Geometry: final body of the model. Coordinates: model frame, mm. A direction names the side the tool comes from. Coordinates: 2 decimals unless noted, no trailing zeros. Loops run counter-clockwise (first coordinate to the right, second up) from the corner with the lowest first, then second, coordinate; pieces in that order, holes last. Notation, with made-up numbers: (26, 21) -> (44, 21) arc R28 cw to (44, 39) -> close; hole circle Ø8 at (-19, 54). An arc over 180 degrees is marked (long way). One line per item, written item: value. Start each with the question number.
Item 1: Ray query, probe 1 along Y at (x, z) = (55, -4.6); probe 2 along Y at (x, z) = (5.5, 6). Return the intervals inside material, ascending. Write a range as from..to.
Item 2: Set-up query: faces 4 (the cylindrical face through (-2.708, 64.086, -13.412)), 5 (the flat face through (-4, 1.5, -13)). Return all of +Z, -Z, +X, -X, +Y, -Y with unobstructed straight access to the full face (end or side cutting, diameter ignored); none if empty.
Item 3: Section query C-C on z = -3. Give the number of separate pieces and of enclosed holes in the cut face, then the cut area to 3 significant figures.
Item 4: Mould query, pull axis Y, two halves, no side actions, for faces 1 (the cylindrical face through (56.6, 30.1, -8.2)), 2 (the flat face through (30, -7.5, -5)), 3 (the flat face through (55, 55, -16.37)). Classes: +Y half, -Y half, draft (parallel to the pull), parting line (faces both ways), or undercut.
Item 5: Contact query for flat-ended pins moving along their axis: pin 1 Ø1 at (x, z) = (64, -13) entering from -Y; pin 2 Ø4.5 at (x, y) = (54, 55.5) entering from +Z; pin 3 Ø1.8 at (x, z) = (-5, -13) entering from +Y; pin 4 Ø5 at (x, z) = (64, -8) entering from +Y. Output: stop coordinate, or through.
Item 6: Section query D-D on z = 2.5. Return loops of the section in (x, y), then the cut area to 3 significant figures.
Item 7: Section query A-A on x = 20. Return loops of the section in (y, z), then the cut area to 3 significant figures.
from build123d import *

# Parameters (mm, degrees)
SIDES_START         = -14.970203
SIDES_DEPTH         = 21.970205
BOSS_EXTRUDE2_START = -16.370201
SKETCH1_3_R         = 1.6
BOSS_EXTRUDE2_DEPTH = 1.4
BOSS_EXTRUDE3_START = -16.370203
SKETCH1_4_R         = 1.6
BOSS_EXTRUDE3_DEPTH = 6.000003
BOSS_EXTRUDE4_START = -1.619402
SKETCH1_5_R         = 4.998410694
SKETCH1_5_R_2       = 5.00000078
SKETCH1_5_R_3       = 4.998409474
SKETCH1_5_R_4       = 2
BOSS_EXTRUDE4_DEPTH = 14.75080016
CUT_EXTRUDE1_START  = -7.619402
SKETCH1_6_R         = 2
CUT_EXTRUDE1_DEPTH  = 6
BOSS_EXTRUDE5_START = -1.619402
SKETCH2_R           = 1.6
SKETCH2_W           = 2.2
SKETCH2_H           = 10
BOSS_EXTRUDE5_DEPTH = 13.350799067
BOSS_EXTRUDE6_START = -14.9702
SKETCH2_3_W         = 2.2
SKETCH2_3_H         = 10
BOSS_EXTRUDE6_DEPTH = 19.9702
CUT_EXTRUDE2_START  = -3e-06
CUT_EXTRUDE2_DEPTH  = 23.370208


with BuildPart() as part:
    # Sketch1 → sides (new body)
    with BuildSketch(Plane.XY.offset(SIDES_START)):
        with BuildLine():
            ThreePointArc((-7.5, 62.5), (-6.035533906, 66.035533906), (-2.5, 67.5))
            Line((-2.5, 67.5), (62.5, 67.5))
            ThreePointArc((62.5, 67.5), (66.035533906, 66.035533906), (67.5, 62.5))
            Line((67.5, 62.5), (67.5, -2.5))
            ThreePointArc((67.5, -2.5), (66.035533906, -6.035533906), (62.5, -7.5))
            Line((62.5, -7.5), (-2.5, -7.5))
            ThreePointArc((-2.5, -7.5), (-6.035533906, -6.035533906), (-7.5, -2.5))
            Line((-7.5, -2.5), (-7.5, 62.5))
        make_face()
        with BuildLine():
            ThreePointArc((66, 62.5), (64.974873734, 64.974873734), (62.5, 66))
            Line((62.5, 66), (61, 66))
            Line((61, 66), (-1, 66))
            Line((-1, 66), (-2.5, 66))
            ThreePointArc((-2.5, 66), (-4.974873734, 64.974873734), (-6, 62.5))
            Line((-6, 62.5), (-6, 61.010980342))
            Line((-6, 61.010980342), (-6, -1))
            Line((-6, -1), (-6, -2.5))
            ThreePointArc((-6, -2.5), (-4.974873734, -4.974873734), (-2.5, -6))
            Line((-2.5, -6), (-1, -6))
            Line((-1, -6), (61, -6))
            Line((61, -6), (62.5, -6))
            ThreePointArc((62.5, -6), (64.974873734, -4.974873734), (66, -2.5))
            Line((66, -2.5), (66, -1))
            Line((66, -1), (66, 61.010980342))
            Line((66, 61.010980342), (66, 62.5))
        make_face(mode=Mode.SUBTRACT)
    extrude(amount=SIDES_DEPTH)

    # Sketch1<3> → Boss-Extrude2 (add)
    with BuildSketch(Plane.XY.offset(BOSS_EXTRUDE2_START)):
        with BuildLine():
            Line((67.5, 62.5), (67.5, -2.5))
            ThreePointArc((67.5, -2.5), (66.035533906, -6.035533906), (62.5, -7.5))
            Line((62.5, -7.5), (-2.5, -7.5))
            ThreePointArc((-2.5, -7.5), (-6.035533906, -6.035533906), (-7.5, -2.5))
            Line((-7.5, -2.5), (-7.5, 62.5))
            ThreePointArc((-7.5, 62.5), (-6.035533906, 66.035533906), (-2.5, 67.5))
            Line((-2.5, 67.5), (62.5, 67.5))
            ThreePointArc((62.5, 67.5), (66.035533906, 66.035533906), (67.5, 62.5))
        make_face()
        with Locations((-2.5, 62.5)):
            Circle(SKETCH1_3_R, mode=Mode.SUBTRACT)
        with Locations((62.5, 62.5)):
            Circle(SKETCH1_3_R, mode=Mode.SUBTRACT)
        with Locations((-2.5, -2.5)):
            Circle(SKETCH1_3_R, mode=Mode.SUBTRACT)
        with Locations((62.5, -2.5)):
            Circle(SKETCH1_3_R, mode=Mode.SUBTRACT)
    extrude(amount=BOSS_EXTRUDE2_DEPTH)

    # Sketch1<4> → Boss-Extrude3 (add)
    # profile 1 of 4: a face of its own
    with BuildSketch(Plane.XY.offset(BOSS_EXTRUDE3_START)):
        with BuildLine():
            ThreePointArc((66, 62.5), (64.974873734, 64.974873734), (62.5, 66))
            Line((62.5, 66), (58.5, 66))
            Line((58.5, 66), (58.5, 62.5))
            ThreePointArc((58.5, 62.5), (59.671572875, 59.671572875), (62.5, 58.5))
            Line((62.5, 58.5), (66, 58.5))
            Line((66, 58.5), (66, 62.5))
        make_face()
        with Locations((62.5, 62.5)):
            Circle(SKETCH1_4_R, mode=Mode.SUBTRACT)
    # profile 2 of 4: a face of its own
    with BuildSketch(Plane.XY.offset(BOSS_EXTRUDE3_START)):
        with BuildLine():
            Line((1.5, 62.5), (1.5, 66))
            Line((1.5, 66), (-2.5, 66))
            ThreePointArc((-2.5, 66), (-4.974873734, 64.974873734), (-6, 62.5))
            Line((-6, 62.5), (-6, 58.5))
            Line((-6, 58.5), (-2.5, 58.5))
            ThreePointArc((-2.5, 58.5), (0.328427125, 59.671572875), (1.5, 62.5))
        make_face()
        with Locations((-2.5, 62.5)):
            Circle(SKETCH1_4_R, mode=Mode.SUBTRACT)
    # profile 3 of 4: a face of its own
    with BuildSketch(Plane.XY.offset(BOSS_EXTRUDE3_START)):
        with BuildLine():
            Line((66, -2.5), (66, 1.5))
            Line((66, 1.5), (62.5, 1.5))
            ThreePointArc((62.5, 1.5), (59.671572875, 0.328427125), (58.5, -2.5))
            Line((58.5, -2.5), (58.5, -6))
            Line((58.5, -6), (62.5, -6))
            ThreePointArc((62.5, -6), (64.974873734, -4.974873734), (66, -2.5))
        make_face()
        with Locations((62.5, -2.5)):
            Circle(SKETCH1_4_R, mode=Mode.SUBTRACT)
    # profile 4 of 4: a face of its own
    with BuildSketch(Plane.XY.offset(BOSS_EXTRUDE3_START)):
        with BuildLine():
            Line((-2.5, 1.5), (-6, 1.5))
            Line((-6, 1.5), (-6, -2.5))
            ThreePointArc((-6, -2.5), (-4.974873734, -4.974873734), (-2.5, -6))
            Line((-2.5, -6), (1.5, -6))
            Line((1.5, -6), (1.5, -2.5))
            ThreePointArc((1.5, -2.5), (0.328427125, 0.328427125), (-2.5, 1.5))
        make_face()
        with Locations((-2.5, -2.5)):
            Circle(SKETCH1_4_R, mode=Mode.SUBTRACT)
    extrude(amount=BOSS_EXTRUDE3_DEPTH)

    # Sketch1<5> → Boss-Extrude4 (add)
    with BuildSketch(Plane.XY.offset(BOSS_EXTRUDE4_START)):
        with Locations((55.001589559, 4.998410441)):
            Circle(SKETCH1_5_R)
        with Locations((54.99999922, 54.99999922)):
            Circle(SKETCH1_5_R_2)
        with Locations((5.00000016, 54.99999922)):
            Circle(SKETCH1_5_R_2)
        with Locations((4.998409221, 4.998409221)):
            Circle(SKETCH1_5_R_3)
        with Locations((4.998409221, 4.998409221)):
            Circle(SKETCH1_5_R_4)
        with Locations((55.001589559, 4.998410441)):
            Circle(SKETCH1_5_R_4)
        with Locations((54.99999922, 54.99999922)):
            Circle(SKETCH1_5_R_4)
        with Locations((5.00000016, 54.99999922)):
            Circle(SKETCH1_5_R_4)
    extrude(amount=-BOSS_EXTRUDE4_DEPTH)

    # Sketch1<6> → Cut-Extrude1 (cut)
    with BuildSketch(Plane.XY.offset(CUT_EXTRUDE1_START)):
        with Locations((4.998409221, 4.998409221)):
            Circle(SKETCH1_6_R)
        with Locations((55.001589559, 4.998410441)):
            Circle(SKETCH1_6_R)
        with Locations((54.99999922, 54.99999922)):
            Circle(SKETCH1_6_R)
        with Locations((5.00000016, 54.99999922)):
            Circle(SKETCH1_6_R)
    extrude(amount=CUT_EXTRUDE1_DEPTH, mode=Mode.SUBTRACT)

    # Sketch2 → Boss-Extrude5 (add)
    # profile 1 of 4: a face of its own
    with BuildSketch(Plane.XY.offset(BOSS_EXTRUDE5_START)):
        with BuildLine():
            ThreePointArc((-1.6, 25), (3.4, 30), (-1.6, 35))
            Line((-1.6, 35), (-3.8, 35))
            Line((-3.8, 35), (-3.8, 25))
            Line((-3.8, 25), (-1.6, 25))
        make_face()
        with Locations((-1.6, 30)):
            Circle(SKETCH2_R, mode=Mode.SUBTRACT)
    # profile 2 of 4: a face of its own
    with BuildSketch(Plane.XY.offset(BOSS_EXTRUDE5_START)):
        with Locations((-4.9, 30)):
            Rectangle(SKETCH2_W, SKETCH2_H)
    # profile 3 of 4: a face of its own
    with BuildSketch(Plane.XY.offset(BOSS_EXTRUDE5_START)):
        with BuildLine():
            Line((63.8, 35), (61.6, 35))
            ThreePointArc((61.6, 35), (56.6, 30), (61.6, 25))
            Line((61.6, 25), (63.8, 25))
            Line((63.8, 25), (63.8, 35))
        make_face()
        with Locations((61.6, 30)):
            Circle(SKETCH2_R, mode=Mode.SUBTRACT)
    # profile 4 of 4: a face of its own
    with BuildSketch(Plane.XY.offset(BOSS_EXTRUDE5_START)):
        with Locations((64.9, 30)):
            Rectangle(SKETCH2_W, SKETCH2_H)
    extrude(amount=-BOSS_EXTRUDE5_DEPTH)

    # Sketch2<3> → Boss-Extrude6 (add)
    with BuildSketch(Plane.XY.offset(BOSS_EXTRUDE6_START)):
        with Locations((-4.9, 30)):
            Rectangle(SKETCH2_3_W, SKETCH2_3_H)
        with Locations((64.9, 30)):
            Rectangle(SKETCH2_3_W, SKETCH2_3_H)
    extrude(amount=BOSS_EXTRUDE6_DEPTH)

    # Sketch3 → Cut-Extrude2 (cut)
    with BuildSketch(Plane(origin=(0, 7.16e-07, -16.370202778), x_dir=(1, 0, 0), z_dir=(4.178627238637217e-15, -4.371140900000003e-08, 0.999999999999999)).offset(CUT_EXTRUDE2_START)):
        with BuildLine():
            Line((23.053327071, 25.897848181), (13.305327071, 25.897848181))
            ThreePointArc((13.305327071, 25.897848181), (11.184006728, 25.019168525), (10.305327071, 22.897848181))
            Line((10.305327071, 22.897848181), (10.305327071, 3.06e-07))
            ThreePointArc((10.305327071, 3.06e-07), (11.184006728, -2.121320038), (13.305327071, -2.999999694))
            Line((13.305327071, -2.999999694), (23.053327071, -2.999999694))
            ThreePointArc((23.053327071, -2.999999694), (25.174647415, -2.121320038), (26.053327071, 3.06e-07))
            Line((26.053327071, 3.06e-07), (26.053327071, 22.897848181))
            ThreePointArc((26.053327071, 22.897848181), (25.174647415, 25.019168525), (23.053327071, 25.897848181))
        make_face()
    extrude(amount=CUT_EXTRUDE2_DEPTH, mode=Mode.SUBTRACT)


solid = part.part
Reply:
1. probe 1: y = -7.5..-6, 0..3, 7..10, 50..53, 57..60, 66..67.5
1. probe 2: y = -7.5..-6, 66..67.5
2. face 4: +Z, -Z
2. face 5: +Z
3. separate pieces: 5
3. enclosed holes: 7
3. area: 844 mm²
4. face 1: undercut
4. face 2: -Y half
4. face 3: draft
5. pin 1: stops at y = -7.4
5. pin 2: stops at z = -1.62
5. pin 3: stops at y = 67.24
5. pin 4: stops at y = 67.5
6. outline: (-7.5, -2.5) arc R5 ccw to (-2.5, -7.5) -> (62.5, -7.5) arc R5 ccw to (67.5, -2.5) -> (67.5, 62.5) arc R5 ccw to (62.5, 67.5) -> (-2.5, 67.5) arc R5 ccw to (-7.5, 62.5) -> close; hole (-6, -2.5) arc R3.5 ccw to (-2.5, -6) -> (62.5, -6) arc R3.5 ccw to (66, -2.5) -> (66, 25) -> (63.8, 25) -> (63.8, 35) -> (66, 35) -> (66, 62.5) arc R3.5 ccw to (62.5, 66) -> (-2.5, 66) arc R3.5 ccw to (-6, 62.5) -> (-6, 35) -> (-3.8, 35) -> (-3.8, 25) -> (-6, 25) -> close
6. area: 474 mm²
7. outline: (-7.5, -16.37) -> (-3, -16.37) -> (-3, -14.97) -> (-6, -14.97) -> (-6, 7) -> (-7.5, 7) -> close; (25.9, -16.37) -> (67.5, -16.37) -> (67.5, 7) -> (66, 7) -> (66, -14.97) -> (25.9, -14.97) -> close
7. area: 130 mm²
